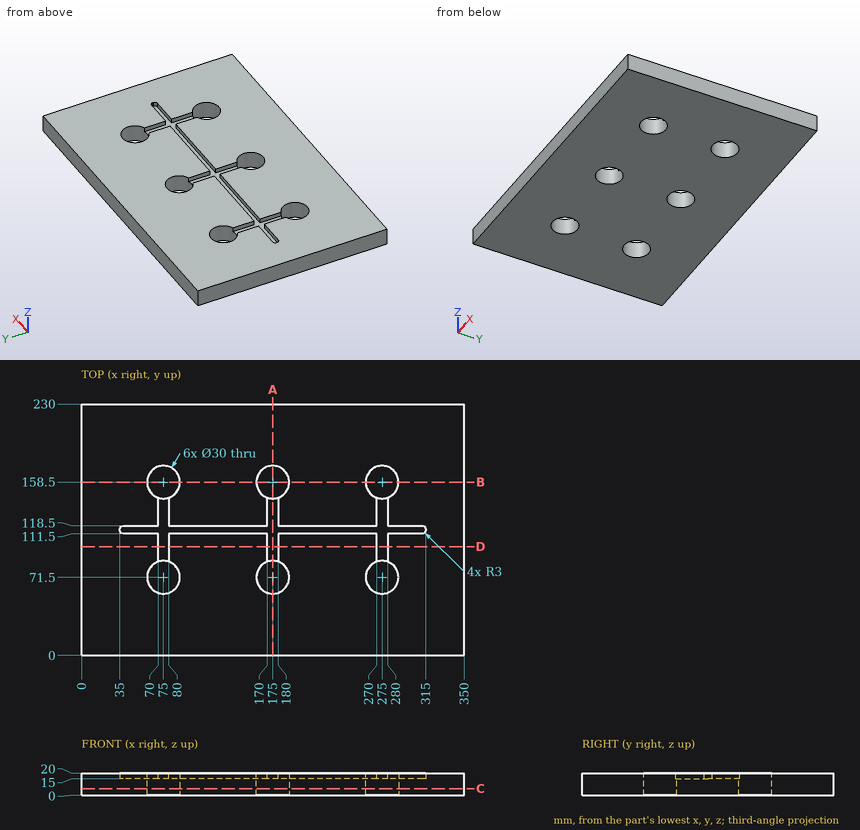
Here's the drawing with two shaded views (mm, measured from the low corner). I have some questions. Give positions to 0.01 mm unless a question says otherwise; leave off trailing zeros. Loops run counter-clockwise (first coordinate to the right, second up) from the corner with the lowest first, then second, coordinate; pieces in that order, holes last. Notation, with made-up numbers: (33, -11) - (48, -11) arc R26 ccw to (48, 7) - close; hole circle Ø3 at (-37, 9). An arc over 180 degrees is marked (long way). One line per item, written item: value.
(1) If we section it at D-D, the plane y = 99.5: List the corners of the cut face in (x, z) for me, plus the area to 3 significant figures.
Verdict:
outline: (0, 0) - (350, 0) - (350, 20) - (280, 20) - (280, 15) - (270, 15) - (270, 20) - (180, 20) - (180, 15) - (170, 15) - (170, 20) - (80, 20) - (80, 15) - (70, 15) - (70, 20) - (0, 20) - close
area: 6,850 mm^2
(2) If we section it at B-B, the plane y = 158.5: List the corners of the cut face in (x, z) for me.
Verdict:
outline: (0, 0) - (60, 0) - (60, 20) - (0, 20) - close; (90, 0) - (160, 0) - (160, 20) - (90, 20) - close; (190, 0) - (260, 0) - (260, 20) - (190, 20) - close; (290, 0) - (350, 0) - (350, 20) - (290, 20) - close
(3) I need wall thicknesses on line 1 along X through (y, z) = (71.5, 5.75); line 2 along Y through (x, z) = (175, 13); line 3 along Y through (x, z) = (275, 15.5). Which ranges of each line are inside material? Lowest first, please.
Verdict:
line 1: 0 to 60, 90 to 160, 190 to 260, 290 to 350
line 2: 0 to 56.5, 86.5 to 143.5, 173.5 to 230
line 3: 0 to 56.5, 173.5 to 230
(4) I'm going to push flat-ended pins straight in: pin 1 (4 mm diameter, centred on y = 135, z = 18.5, fed in from -X); pin 2 (24 mm diameter, centred on x = 175, y = 71.5, fed in from +Z). Where does each tip first touch, or does it pass through?
Verdict:
pin 1: x = 0
pin 2: through
(5) If we section it at A-A, the plane x = 175: List the corners of the cut face in (y, z) for me.
Verdict:
outline: (0, 0) - (56.5, 0) - (56.5, 20) - (0, 20) - close; (86.5, 0) - (143.5, 0) - (143.5, 15) - (86.5, 15) - close; (173.5, 0) - (230, 0) - (230, 20) - (173.5, 20) - close
(6) If we section it at C-C, the plane z = 6: List the corners of the cut face in (x, y) for me.
Verdict:
outline: (0, 0) - (350, 0) - (350, 230) - (0, 230) - close; hole circle Ø30 at (75, 71.5); hole circle Ø30 at (75, 158.5); hole circle Ø30 at (175, 71.5); hole circle Ø30 at (175, 158.5); hole circle Ø30 at (275, 71.5); hole circle Ø30 at (275, 158.5)
